Model file for the job. Use its own axes, mm. A direction names the side the tool comes from. Give positions to 0.01 mm unless a question says otherwise; leave off trailing zeros. Loops run counter-clockwise (first coordinate to the right, second up) from the corner with the lowest first, then second, coordinate; pieces in that order, holes last. Notation, with made-up numbers: (-16.75, 53) - (-2.75, 53) arc R16 ccw to (-2.75, 57) - close; hole circle Ø10 at (5.25, -34). An arc over 180 degrees is marked (long way). Use a Markdown table: item, result.
from build123d import *

# Parameters (mm, degrees)
BOX001_W     = 4
BOX001_H     = 11
BOX001_DEPTH = 12
BOX002_W     = 4
BOX002_H     = 11
BOX002_DEPTH = 12
BOX_W        = 4
BOX_H        = 11
BOX_DEPTH    = 12
BOX003_W     = 45
BOX003_H     = 21
BOX003_DEPTH = 10


with BuildPart() as cube001:
    # Box001 → Box001 (new body)
    with BuildSketch(Plane(origin=(15, 0, 0), x_dir=(1, 0, 0), z_dir=(0, 0, 1))):
        with Locations((2, 5.5)):
            Rectangle(BOX001_W, BOX001_H)
    extrude(amount=BOX001_DEPTH)


with BuildPart() as cube002:
    # Box002 → Box002 (new body)
    with BuildSketch(Plane(origin=(30, 0, 0), x_dir=(1, 0, 0), z_dir=(0, 0, 1))):
        with Locations((2, 5.5)):
            Rectangle(BOX002_W, BOX002_H)
    extrude(amount=BOX002_DEPTH)


with BuildPart() as fusion:
    # Box → Box (new body)
    with BuildSketch(Plane.XY):
        with Locations((2, 5.5)):
            Rectangle(BOX_W, BOX_H)
    extrude(amount=BOX_DEPTH)

    # Fusion: union Cube001, Cube002
    add(cube001.part)
    add(cube002.part)


with BuildPart() as fusion_1:
    # Fusion placement: moved
    add(fusion.part.moved(Location((5, 5, 3))))


with BuildPart() as cut:
    # Box003 → Box003 (new body)
    with BuildSketch(Plane.XY):
        with Locations((22.5, 10.5)):
            Rectangle(BOX003_W, BOX003_H)
    extrude(amount=BOX003_DEPTH)

    # Cut: cut Fusion
    add(fusion_1.part, mode=Mode.SUBTRACT)


solid = cut.part
(1) Slice it at B-B, the plane y = 9. Write the cut outline in (x, z).
Computed:
| item | result |
|---|---|
| outline | (0, 0) - (45, 0) - (45, 10) - (39, 10) - (39, 3) - (35, 3) - (35, 10) - (24, 10) - (24, 3) - (20, 3) - (20, 10) - (9, 10) - (9, 3) - (5, 3) - (5, 10) - (0, 10) - close |
(2) 3-axis set-ups, long thin cutter, end or side, ignore diameter. For faces 5 (the flat face through (22, 0, 5)), 6 (the flat face through (24, 10, 6)): which of +Z, -Z, +X, -X, +Y, -Y reach the whole face in a straight line?
Computed:
| item | result |
|---|---|
| face 5 | +Z, -Z, +X, -X, -Y |
| face 6 | +Z |
(3) Drill centre lines: probe 1 along X at (y, z) = (12, 8); probe 2 along Y at (x, z) = (36, 5.75); probe 3 along Z at (x, y) = (37.5, 10). Where is each one in solid material? Low to high. Write a range as [from, to].
Computed:
| item | result |
|---|---|
| probe 1 | [0, 5], [9, 20], [24, 35], [39, 45] |
| probe 2 | [0, 5], [16, 21] |
| probe 3 | [0, 3] |
(4) Pin check, flat tip, straight feed: P1, Ø2, axis at x = 7.5, y = 8.5, coming from the +Z side. Stop position of the tip, or through.
Computed:
| item | result |
|---|---|
| P1 | z = 3 |
(5) Slice it at C-C, the plane x = 8. Write the cut outline in (y, z), plus the area to 3 significant figures.
Computed:
| item | result |
|---|---|
| outline | (0, 0) - (21, 0) - (21, 10) - (16, 10) - (16, 3) - (5, 3) - (5, 10) - (0, 10) - close |
| area | 133 mm² |
(6) Mould opens along Y. For faces 1 (the flat face through (9, 10, 6)), 2 (the flat face through (22, 11, 0)), 3 (the flat face through (22, 21, 5)), 4 (the flat face through (7, 16, 6)) say: pulls with the +Y half, pulls with the -Y half, needs draft (parallel to the pull), parting line crosses it, or undercut.
Computed:
| item | result |
|---|---|
| face 1 | undercut |
| face 2 | needs draft |
| face 3 | pulls with the +Y half |
| face 4 | undercut |
(7) Slice it at A-A, the plane z = 7.25. Write the cut outline in (x, y), plus the area to 3 significant figures.
Computed:
| item | result |
|---|---|
| outline | (0, 0) - (45, 0) - (45, 21) - (0, 21) - close; hole (5, 5) - (9, 5) - (9, 16) - (5, 16) - close; hole (20, 5) - (24, 5) - (24, 16) - (20, 16) - close; hole (35, 5) - (39, 5) - (39, 16) - (35, 16) - close |
| area | 813 mm² |
